The model under review builds one solid part; all positions refer to its coordinate system, in mm. A direction names the side the tool comes from. Give positions to 0.01 mm unless a question says otherwise; leave off trailing zeros. Write each loop counter-clockwise with the first axis right and the second up, starting at its lowest first coordinate (ties: lowest second). Pieces come first, ordered by that corner, then holes. Notation, with made-up numbers: (21, 65) -> (61, 65) arc R17 cw to (61, 88) -> close; hole circle Ø2 at (-31, 38). An arc over 180 degrees is marked (long way). Use CSV: the item, a comma, the result in double quotes.
```python
from build123d import *

# Parameters (mm, degrees)
F0_W     = 88
F0_H     = 100
F2_DEPTH = 3
F1_W     = 88
F1_H     = 100
F1_W_2   = 82
F1_H_2   = 94
F3_DEPTH = 70
F4_R     = 3
F5_R     = 1.5
F6_DEPTH = 25
F8_DEPTH = 25


with BuildPart() as f2:
    # F0 (on Top) → F2 (new body)
    with BuildSketch(Plane.XY):
        with Locations((8.683464, 2.622797)):
            Rectangle(F0_W, F0_H)
    extrude(amount=-F2_DEPTH)

    # F1 (on face) → F3 (join)
    with BuildSketch(Plane.XY):
        with Locations((8.683464, 2.622797)):
            Rectangle(F1_W, F1_H)
        with Locations((8.683464, 2.622797)):
            Rectangle(F1_W_2, F1_H_2, mode=Mode.SUBTRACT)
    extrude(amount=F3_DEPTH)

    # F4
    f4_edges = [f2.edges().sort_by_distance(p)[0] for p in [
        (-35.316536, 2.622797, -3),
        (8.683464, 52.622797, -3),
        (8.683464, -47.377203, -3),
        (52.683464, 2.622797, -3),
    ]]
    fillet(f4_edges, radius=F4_R)

    # F5 (on face) → F6 (cut)
    with BuildSketch(Plane(origin=(-35.316536, 0, 0), x_dir=(0, -1, 0), z_dir=(-1, 0, 0))):
        with Locations((-46.622797, 67)):
            Circle(F5_R)
        with Locations((41.377203, 67)):
            Circle(F5_R)
    extrude(amount=-F6_DEPTH, mode=Mode.SUBTRACT)

    # F7 (on face) → F8 (cut)
    with BuildSketch(Plane.YZ.offset(52.683464)):
        with BuildLine():
            ThreePointArc((2.622797, 68.5), (1.562137, 65.93934), (4.122797, 67))
            ThreePointArc((4.122797, 67), (3.683457, 68.06066), (2.622797, 68.5))
        make_face()
    extrude(amount=-F8_DEPTH, mode=Mode.SUBTRACT)


solid = f2.part
```
Q1. Insertion check: pin 1 (6 mm diameter, centred on x = 38, y = -24, fed in from +Z). The pin has a flat end and moves straight along its axis. Give the tip position at first contact, or say it passes through.
Derived:
pin 1,"stops at z = 0"
Q2. Machinability: for faces 5 (the flat face through (-34, 3, 70)), 6 (the flat face through (8, 49.623, 35)), which of the approach directions +Z, -Z, +X, -X, +Y, -Y give a long, thin tool a straight path to every point of the face, cutting with its end or side? Answer none if there is none.
Derived:
face 5,"+Z, +X, -X, +Y, -Y"
face 6,"+Z"
Q3. To check wall thickness, follow probe 1 along Y at (x, z) = (-34, 67); probe 2 along Y at (x, z) = (11, 10.5); probe 3 along X at (y, z) = (-17.5, 45). State the ranges of each line that lie inside material, in increasing order.
Derived:
probe 1,"y = -47.38 to -42.88, -39.88 to 45.12, 48.12 to 52.62"
probe 2,"y = -47.38 to -44.38, 49.62 to 52.62"
probe 3,"x = -35.32 to -32.32, 49.68 to 52.68"
Q4. Consider section A-A (z = 26). Write out the cut boundary in (x, y), then the cut area to 3 significant figures.
Derived:
outline,"(-35.32, -47.38) -> (52.68, -47.38) -> (52.68, 52.62) -> (-35.32, 52.62) -> close; hole (-32.32, -44.38) -> (49.68, -44.38) -> (49.68, 49.62) -> (-32.32, 49.62) -> close"
area,"1,090 mm2"
Q5. Consider section B-B (x = 18). Write out the cut boundary in (y, z).
Derived:
outline,"(-47.38, 0) arc R3 ccw to (-44.38, -3) -> (49.62, -3) arc R3 ccw to (52.62, 0) -> (52.62, 70) -> (49.62, 70) -> (49.62, 0) -> (-44.38, 0) -> (-44.38, 70) -> (-47.38, 70) -> close"
Q6. Consider section C-C (y = -34.5). Write out the cut boundary in (x, z), then the cut area to 3 significant figures.
Derived:
outline,"(-35.32, 0) arc R3 ccw to (-32.32, -3) -> (49.68, -3) arc R3 ccw to (52.68, 0) -> (52.68, 70) -> (49.68, 70) -> (49.68, 0) -> (-32.32, 0) -> (-32.32, 70) -> (-35.32, 70) -> close"
area,"680 mm2"
Q7. The part is to be moulded in two halves that separate along Z. For faces 1 (the cylindrical face through (-33.84, -39.88, 67.07)), 2 (the cylindrical face through (9.3, -46.52, -2.1)), 3 (the flat face through (8, 3, 0)), 4 (the cylindrical face through (-33.84, 48.12, 67.07)), say which applies: pulls with the +Z half, pulls with the -Z half, needs draft (parallel to the pull), parting line crosses it, or undercut.
Derived:
face 1,"undercut"
face 2,"pulls with the -Z half"
face 3,"pulls with the +Z half"
face 4,"undercut"
